Input: part model. Units: mm. Frame: model coordinates. A direction names the side the tool comes from. Coordinates: 2 decimals unless noted, no trailing zeros. Loops run counter-clockwise (first coordinate to the right, second up) from the corner with the lowest first, then second, coordinate; pieces in that order, holes last.
```python
from build123d import *

# Parameters (mm, degrees)
CROQUIS1_R                                           = 42.75
SALIENTE_EXTRUIR1_DEPTH                              = 3.5
REFRENTADO_PARA_TORNILLO_CON_CABEZA_TRON_D           = 3.4
REFRENTADO_PARA_TORNILLO_CON_CABEZA_TRON_DEPTH       = 20
REFRENTADO_PARA_TORNILLO_CON_CABEZA_TRON_CBORE_D     = 7
REFRENTADO_PARA_TORNILLO_CON_CABEZA_TRON_CBORE_DEPTH = 2.4
REFRENTADO_PARA_TORNILLO_CON_CABEZA_TRON_TIP         = 1.021463052
CROQUIS4_R                                           = 22.5
SALIENTE_EXTRUIR2_DEPTH                              = 5
CROQUIS5_R                                           = 27.5
SALIENTE_EXTRUIR3_DEPTH                              = 15


with BuildPart() as part:
    # Croquis1 → Saliente-Extruir1 (new, symmetric)
    with BuildSketch(Plane(origin=(0, 0, 0), x_dir=(0, 0, -1), z_dir=(1, 0, 0))):
        Circle(CROQUIS1_R)
    extrude(amount=SALIENTE_EXTRUIR1_DEPTH, both=True)

    # Refrentado para tornillo con cabeza troncocónica de M31
    with Locations(Plane(origin=(3.5, 0, 0), x_dir=(0, 0, -1), z_dir=(1, 0, 0))):
        with Locations((0, 35), (24.748737342, 24.748737342), (35, 0), (24.748737342, -24.748737342), (0, -35), (-24.748737342, -24.748737342), (-35, 0), (-24.748737342, 24.748737342)):
            CounterBoreHole(REFRENTADO_PARA_TORNILLO_CON_CABEZA_TRON_D / 2, REFRENTADO_PARA_TORNILLO_CON_CABEZA_TRON_CBORE_D / 2, REFRENTADO_PARA_TORNILLO_CON_CABEZA_TRON_CBORE_DEPTH, depth=REFRENTADO_PARA_TORNILLO_CON_CABEZA_TRON_DEPTH)
            with Locations((0, 0, -(REFRENTADO_PARA_TORNILLO_CON_CABEZA_TRON_DEPTH + REFRENTADO_PARA_TORNILLO_CON_CABEZA_TRON_TIP / 2))):  # 118° drill point
                Cone(0, REFRENTADO_PARA_TORNILLO_CON_CABEZA_TRON_D / 2, REFRENTADO_PARA_TORNILLO_CON_CABEZA_TRON_TIP, mode=Mode.SUBTRACT)

    # Croquis4 → Saliente-Extruir2 (add)
    with BuildSketch(Plane(origin=(3.5, 0, 0), x_dir=(0, 0, -1), z_dir=(1, 0, 0))):
        Circle(CROQUIS4_R)
    extrude(amount=SALIENTE_EXTRUIR2_DEPTH)

    # Croquis5 → Saliente-Extruir3 (add)
    with BuildSketch(Plane(origin=(8.5, 0, 0), x_dir=(0, 0, -1), z_dir=(1, 0, 0))):
        Circle(CROQUIS5_R)
    extrude(amount=SALIENTE_EXTRUIR3_DEPTH)


solid = part.part
```
Item 1: Line query: L1, parallel to X at y = -18.5, z = -18; L2, parallel to Z at x = 2.25, y = 24; L3, parallel to X at y = -11.5, z = -36. Output: solid intervals per line, ascending.
Result:
L1: x = -3.5 to 3.5, 8.5 to 23.5
L2: z = -35.38 to -28.17, -21.33 to 21.33, 28.17 to 35.38
L3: x = -3.5 to 3.5
Item 2: Mould query, pull axis Z, two halves, no side actions, for faces 1 (the face through (15.895, -26.846, 5.961)), 2 (the face through (2.3, -2.1, -32.2)), 3 (the face through (-3.5, 1, 1)). Classes: +Z half, -Z half, draft (parallel to the pull), parting line (faces both ways), or undercut.
Result:
face 1: parting line
face 2: undercut
face 3: draft
Item 3: Contact query for flat-ended pins moving along their axis: P1, Ø8, axis at x = 15, y = -25, coming from the +Z side; P2, Ø6, axis at x = 10.5, z = -18, coming from the -Y side; P3, Ø2, axis at y = 0.5, z = 35, coming from the +X side; P4, Ø7.5, axis at y = 23.5, z = 24.5, coming from the +X side. Output: stop coordinate, or through.
Result:
P1: stops at z = 17.76
P2: stops at y = -23.05
P3: passes through
P4: stops at x = 3.5
Item 4: Section query A-A (z = 0). Output: boundary loops of the cut face in (x, y).
Result:
outline: (-3.5, -42.75) - (3.5, -42.75) - (3.5, -38.5) - (1.1, -38.5) - (1.1, -36.7) - (-3.5, -36.7) - close; (-3.5, -33.3) - (1.1, -33.3) - (1.1, -31.5) - (3.5, -31.5) - (3.5, -22.5) - (8.5, -22.5) - (8.5, -27.5) - (23.5, -27.5) - (23.5, 27.5) - (8.5, 27.5) - (8.5, 22.5) - (3.5, 22.5) - (3.5, 31.5) - (1.1, 31.5) - (1.1, 33.3) - (-3.5, 33.3) - close; (-3.5, 36.7) - (1.1, 36.7) - (1.1, 38.5) - (3.5, 38.5) - (3.5, 42.75) - (-3.5, 42.75) - close
Item 5: Reachability of faces 4 (the face through (2.317, -24.595, -21.252)), 5 (the face through (-1.23, -36.66, -0.37)) from +Z, -Z, +X, -X, +Y, -Y: full face, straight path, thin tool, end or side. Return the list, or none.
Result:
face 4: +X
face 5: +X, -X
Item 6: Section query C-C (y = -35). Output: boundary loops of the cut face in (x, z).
Result:
outline: (-3.5, -24.55) - (3.5, -24.55) - (3.5, -3.5) - (1.1, -3.5) - (1.1, -1.7) - (-3.5, -1.7) - close; (-3.5, 1.7) - (1.1, 1.7) - (1.1, 3.5) - (3.5, 3.5) - (3.5, 24.55) - (-3.5, 24.55) - close
